from build123d import *

# Parameters (mm, degrees)
F0_R     = 2.5
F0_W     = 10
F0_H     = 15
F1_DEPTH = 2.5
F3_W     = 5
F3_H     = 15
F4_DEPTH = 25


with BuildPart() as f1:
    # F0 (on Top) → F1 (new body)
    with BuildSketch(Plane.XY):
        with BuildLine():
            Line((0, 15), (0, 0))
            Line((0, 0), (48, 0))
            Line((48, 0), (48, 15))
            Line((48, 15), (27.9, 15))
            ThreePointArc((27.9, 15), (27.192893, 14.707107), (26.9, 14))
            Line((26.9, 14), (26.9, 8))
            ThreePointArc((26.9, 8), (26.607107, 7.292893), (25.9, 7))
            Line((25.9, 7), (22.1, 7))
            ThreePointArc((22.1, 7), (21.392893, 7.292893), (21.1, 8))
            Line((21.1, 8), (21.1, 14))
            ThreePointArc((21.1, 14), (20.807107, 14.707107), (20.1, 15))
            Line((20.1, 15), (0, 15))
        make_face()
        with Locations((7.45, 7.5)):
            Circle(F0_R, mode=Mode.SUBTRACT)
        with Locations((37.45, 7.5)):
            Circle(F0_R, mode=Mode.SUBTRACT)
        with Locations((53, 7.5)):
            Rectangle(F0_W, F0_H)
    extrude(amount=F1_DEPTH)

    # F3 (on offset) → F4 (join)
    with BuildSketch(Plane.XY.offset(2.5)):
        with Locations((55.5, 7.5)):
            Rectangle(F3_W, F3_H)
    extrude(amount=F4_DEPTH)


solid = f1.part
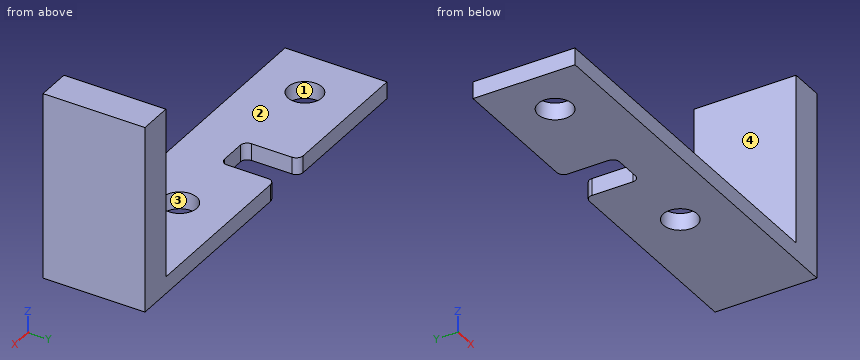
Source: CAD feature listing. Evaluate the final solid. Frame: model axes, mm. Face numbers are marked on the shaded views. Give positions to 0.01 mm unless a question says otherwise; leave off trailing zeros. Order: outer loops, then holes, each group sorted by start corner. A loop starts at its lowest first (then second) coordinate and runs counter-clockwise, first axis right, second up. Notation, with made-up numbers: (-1, 49.25) -> (8, 49.25) arc R15 ccw to (8, 65.25) -> close; hole circle Ø8 at (10.25, -6.5). An arc over 180 degrees is marked (long way). Use a Markdown table: item, result.
1) Section query A-A, the plane x = 7.45. Return the cut outline in (y, z).
Answer list:
| item | result |
|---|---|
| outline | (0, 0) -> (5, 0) -> (5, 2.5) -> (0, 2.5) -> close; (10, 0) -> (15, 0) -> (15, 2.5) -> (10, 2.5) -> close |
2) Section query B-B, the plane y = 12. Return the cut outline in (x, z).
Answer list:
| item | result |
|---|---|
| outline | (0, 0) -> (21.1, 0) -> (21.1, 2.5) -> (0, 2.5) -> close; (26.9, 0) -> (58, 0) -> (58, 27.5) -> (53, 27.5) -> (53, 2.5) -> (26.9, 2.5) -> close |
3) Section query C-C, the plane x = 51. Return the cut outline in (y, z).
Answer list:
| item | result |
|---|---|
| outline | (0, 0) -> (15, 0) -> (15, 2.5) -> (0, 2.5) -> close |
4) Ray query, line 1 along Y through (x, z) = (7.45, 0.75); line 2 along Z through (x, y) = (20, 14); line 3 along X through (y, z) = (13.25, 17.75). Return the intervals inside material, ascending. Write a range as [from, to].
Answer list:
| item | result |
|---|---|
| line 1 | [0, 5], [10, 15] |
| line 2 | [0, 2.5] |
| line 3 | [53, 58] |
5) Section query D-D, the plane z = 13.5. Return the cut outline in (x, y).
Answer list:
| item | result |
|---|---|
| outline | (53, 0) -> (58, 0) -> (58, 15) -> (53, 15) -> close |
6) Mould query, pull axis X, two halves, no side actions, for the marked faces 1, 2, 3 and 4. Classes: +X half, -X half, draft (parallel to the pull), parting line (faces both ways), or undercut.
Answer list:
| item | result |
|---|---|
| face 1 | undercut |
| face 2 | draft |
| face 3 | undercut |
| face 4 | -X half |
7) Contact query for flat-ended pins moving along their axis: P1, Ø2, axis at y = 11.5, z = 1.5, coming from the -X side; P2, Ø4, axis at y = 5.5, z = 6.5, coming from the -X side; P3, Ø3, axis at x = 23.5, z = 2, coming from the +Y side (3 decimals). Output: stop coordinate, or through.
Answer list:
| item | result |
|---|---|
| P1 | x = 0 |
| P2 | x = 53 |
| P3 | y = 7.005 |
